```python
from build123d import *

# Parameters (mm, degrees)
EXTRUDE_2_DEPTH      = 3
EXTRUDE_2_DEPTH_BACK = 3
SKETCH_2_R           = 1.5
EXTRUDE_3_DEPTH      = 30


with BuildPart() as part:
    # Sketch 1 → Extrude 2 (new, two sides: drawn at the far end of the back side and taken through both)
    with BuildSketch(Plane(origin=(0, 0, 0), x_dir=(0, 0, -1), z_dir=(1, 0, 0)).offset(-EXTRUDE_2_DEPTH_BACK)):
        with BuildLine():
            ThreePointArc((10, 0), (7.071067812, 7.071067812), (0, 10))
            Line((0, 10), (0, 2))
            ThreePointArc((0, 2), (1.414213562, 1.414213562), (2, 0))
            ThreePointArc((2, 0), (1.414213562, -1.414213562), (0, -2))
            Line((0, -2), (0, -10))
            ThreePointArc((0, -10), (7.071067812, -7.071067812), (10, 0))
        make_face()
        with BuildLine():
            Line((0, 2), (0, 10))
            ThreePointArc((0, 10), (-10, 0), (0, -10))
            Line((0, -10), (0, -2))
            ThreePointArc((0, -2), (-2, 0), (0, 2))
        make_face()
        with BuildLine():
            Line((10, 0), (10, 10))
            Line((10, 10), (0, 10))
            ThreePointArc((0, 10), (7.071067812, 7.071067812), (10, 0))
        make_face()
        with BuildLine():
            Line((10, -10), (10, 0))
            ThreePointArc((10, 0), (7.071067812, -7.071067812), (0, -10))
            Line((0, -10), (10, -10))
        make_face()
    extrude(amount=EXTRUDE_2_DEPTH + EXTRUDE_2_DEPTH_BACK)

    # Sketch 2 → Extrude 3 (add)
    with BuildSketch(Plane(origin=(0, 0, -10), x_dir=(-1, 0, 0), z_dir=(0, 0, -1))):
        with Locations(Location((0, 0, 0), (0, 0, 270))):
            Circle(SKETCH_2_R)
    extrude(amount=EXTRUDE_3_DEPTH)


solid = part.part
```
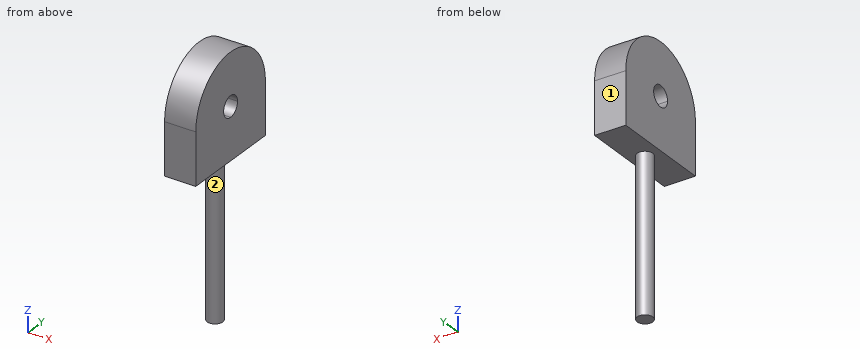
Here's how the part is built. I have some questions about the finished solid (model axes, mm). Face numbers are marked on the shaded views. A direction names the side the tool comes from. Coordinates: 2 decimals unless noted, no trailing zeros. Order: outer loops, then holes, each group sorted by start corner. A loop starts at its lowest first (then second) coordinate and runs counter-clockwise, first axis right, second up.
Item 1: If we section it at B-B, the plane y = -0.75: List the corners of the cut face in (x, z) for me.
Response values:
outline: (-3, -10) - (-1.3, -10) - (-1.3, -40) - (1.3, -40) - (1.3, -10) - (3, -10) - (3, -1.85) - (-3, -1.85) - close; (-3, 1.85) - (3, 1.85) - (3, 9.97) - (-3, 9.97) - close
Item 2: I'm going to push flat-ended pins straight in: pin 1 Ø4 at (y, z) = (1, -32.5) entering from +X; pin 2 Ø3 at (x, z) = (-1, -27) entering from -Y; pin 3 Ø2 at (x, z) = (0, -20.5) entering from +Y. Where does each tip first touch, or does it pass through?
Response values:
pin 1: stops at x = 1.5
pin 2: stops at y = -1.5
pin 3: stops at y = 1.5
Item 3: I need wall thicknesses on probe 1 along Z at (x, y) = (1.7, -1); probe 2 along Y at (x, z) = (0.05, -14.5); probe 3 along Z at (x, y) = (-0.6, -1.25). Which ranges of each line are inside material? Lowest first, please.
Response values:
probe 1: z = -10 to -1.73, 1.73 to 9.95
probe 2: y = -1.5 to 1.5
probe 3: z = -40 to -1.56, 1.56 to 9.92
Item 4: If we section it at D-D, the plane z = -14: List the corners of the cut face in (x, y) for me.
Response values:
outline: circle Ø3 at (0, 0)
Item 5: If we section it at A-A, the plane x = 0: List the corners of the cut face in (y, z) for me.
Response values:
outline: (-10, -10) - (-1.5, -10) - (-1.5, -40) - (1.5, -40) - (1.5, -10) - (10, -10) - (10, 0) arc R10 ccw to (-10, 0) - close; hole circle Ø4 at (0, 0)
Item 6: If we section it at C-C, the plane x = 2.25: List the corners of the cut face in (y, z) for me, then the cut area to 3 significant figures.
Response values:
outline: (-10, -10) - (10, -10) - (10, 0) arc R10 ccw to (-10, 0) - close; hole circle Ø4 at (0, 0)
area: 345 mm2
Item 7: Which directions (+Z, -Z, +X, -X, +Y, -Y) give clear straight access to the entire face, cutting with the end or side of a thin tool? Please do the marked faces 1 and 2.
Response values:
face 1: +Z, -Z, +X, -X, +Y
face 2: -Z
